Input: part model. Units: mm. Frame: model coordinates. A direction names the side the tool comes from. Give positions to 0.01 mm unless a question says otherwise; leave off trailing zeros. Loops run counter-clockwise (first coordinate to the right, second up) from the corner with the lowest first, then second, coordinate; pieces in that order, holes last. Notation, with made-up numbers: M 71.25,11 L 79.25,11 A29 cw 79.25,41 Z; hole C -24.5,31.25 d1. An arc over 180 degrees is marked long. Return JSON: item names as keys, results as strings. Group by question number.
```python
from build123d import *

# Parameters (mm, degrees)
SKETCH1_W                    = 101.6
SKETCH1_H                    = 101.6
EXTRUDE1_DEPTH               = 3.175
SKETCH2_W                    = 101.6
SKETCH2_H                    = 60.96
EXTRUDE2_DEPTH               = 6.35
EXTRUDE3_DEPTH               = 114.990901501
SKETCH4_W                    = 88.9
SKETCH4_H                    = 66.294
EXTRUDE4_DEPTH               = 35.56
SKETCH5_W                    = 27.305
SKETCH5_H                    = 56.134
EXTRUDE5_DEPTH               = 112.536082502
SKETCH6_W                    = 3.175
SKETCH6_H                    = 56.134
EXTRUDE6_DEPTH               = 12.7
SKETCH7_W                    = 8.89
SKETCH7_H                    = 1.27
EXTRUDE7_DEPTH               = 79.375
SKETCH8_W                    = 5.08
SKETCH8_H                    = 35.814
EXTRUDE8_DEPTH               = 19.558
F_5_16_CLEARANCE_HOLE1_D     = 8.4328
F_5_16_CLEARANCE_HOLE1_DEPTH = 12.954
F_5_16_CLEARANCE_HOLE1_TIP   = 2.533468714
EXTRUDE9_DEPTH               = 6.604
F_8_CLEARANCE_HOLE1_D        = 4.4958
LPATTERN1_COUNT              = 2
LPATTERN1_PITCH              = 10.16


with BuildPart() as part:
    # Sketch1 → Extrude1 (new body)
    with BuildSketch(Plane.XY):
        Rectangle(SKETCH1_W, SKETCH1_H)
    extrude(amount=EXTRUDE1_DEPTH)

    # Sketch2 → Extrude2 (add)
    with BuildSketch(Plane.XY.offset(3.175)):
        Rectangle(SKETCH2_W, SKETCH2_H)
    extrude(amount=EXTRUDE2_DEPTH)

    # Sketch3 → Extrude3 (cut, through all)
    with BuildSketch(Plane(origin=(50.8, 0, 0), x_dir=(0, 0, -1), z_dir=(1, 0, 0))):
        Polygon((-9.525, -17.78), (-4.445, -20.712939367), (-4.445, 20.712939367), (-9.525, 17.78), align=None)
    extrude(amount=-EXTRUDE3_DEPTH, mode=Mode.SUBTRACT)

    # Sketch4 → Extrude4 (add)
    with BuildSketch(Plane(origin=(0, 0, 0), x_dir=(-1, 0, 0), z_dir=(0, 0, -1))):
        with Locations((2.54, 0)):
            Rectangle(SKETCH4_W, SKETCH4_H)
    extrude(amount=EXTRUDE4_DEPTH)

    # Sketch5 → Extrude5 (cut, through all)
    with BuildSketch(Plane(origin=(41.91, 0, 0), x_dir=(0, 0, -1), z_dir=(1, 0, 0))):
        with Locations((16.8275, 0)):
            Rectangle(SKETCH5_W, SKETCH5_H)
    extrude(amount=-EXTRUDE5_DEPTH, mode=Mode.SUBTRACT)

    # Sketch6 → Extrude6 (add)
    with BuildSketch(Plane(origin=(0, 0, -3.175), x_dir=(-1, 0, 0), z_dir=(0, 0, -1))):
        with Locations((45.4025, 0)):
            Rectangle(SKETCH6_W, SKETCH6_H)
    extrude(amount=EXTRUDE6_DEPTH)

    # Sketch7 → Extrude7 (cut)
    with BuildSketch(Plane(origin=(41.91, 0, 0), x_dir=(0, 0, -1), z_dir=(1, 0, 0))):
        with Locations((19.05, -28.702)):
            Rectangle(SKETCH7_W, SKETCH7_H)
    extrude(amount=-EXTRUDE7_DEPTH, mode=Mode.SUBTRACT)

    # Sketch8 → Extrude8 (cut)
    with BuildSketch(Plane(origin=(41.91, 0, 0), x_dir=(0, 0, -1), z_dir=(1, 0, 0))):
        with Locations((33.02, 0)):
            Rectangle(SKETCH8_W, SKETCH8_H)
    extrude(amount=-EXTRUDE8_DEPTH, mode=Mode.SUBTRACT)

    # 5/16 Clearance Hole1
    with Locations(Plane(origin=(12.8016, -33.147, -20.066), x_dir=(-1, 0, 0), z_dir=(0, -1, 0))):
        with Locations((0, 0)):
            Hole(F_5_16_CLEARANCE_HOLE1_D / 2, depth=F_5_16_CLEARANCE_HOLE1_DEPTH)
            with Locations((0, 0, -(F_5_16_CLEARANCE_HOLE1_DEPTH + F_5_16_CLEARANCE_HOLE1_TIP / 2))):  # 118° drill point
                Cone(0, F_5_16_CLEARANCE_HOLE1_D / 2, F_5_16_CLEARANCE_HOLE1_TIP, mode=Mode.SUBTRACT)

    # Sketch11 → Extrude9 (add)
    with BuildSketch(Plane.XY.offset(4.445)):
        Polygon((50.8, 0), (50.8, -5.715), (44.45, -5.715), (44.45, 5.715), (50.8, 5.715), align=None)
    extrude9 = extrude(amount=EXTRUDE9_DEPTH)

    # #8 Clearance Hole1 (through all)
    with Locations(Plane(origin=(50.8, 0, 7.62), x_dir=(0, 0, 1), z_dir=(1, 0, 0))):
        with Locations((0, 0)):
            f_8_clearance_hole1 = Hole(F_8_CLEARANCE_HOLE1_D / 2)

    # LPattern1: Extrude9, #8 Clearance Hole1 ×2
    with Locations(*[(-i * LPATTERN1_PITCH, 0, 0) for i in range(1, LPATTERN1_COUNT)]):
        add(extrude9)
        add(f_8_clearance_hole1, mode=Mode.SUBTRACT)


solid = part.part
```
Item 1: Reachability of faces 4 (the face through (0.711, -19.226, 7.021)), 5 (the face through (-1, -40, 3.175)), 6 (the face through (22.352, 0, -33)), 7 (the face through (-2, 28.067, -17)) from +Z, -Z, +X, -X, +Y, -Y: full face, straight path, thin tool, end or side. Return the list, or none.
Item 2: Section C-C, the plane z = 7.62. Return loops of the section in (x, y) (3 decimals).
Item 3: Section A-A, the plane y = 4. Return loops of the section in (x, z) (3 decimals).
Item 4: Pull-direction query (Z, two-part tool) for faces 1 (the face through (3, -29.337, -19)), 2 (the face through (38, 0, 11.049)), 3 (the face through (37, 5.715, 8)); classes: pulls with the +Z half, pulls with the -Z half, needs draft (parallel to the pull), parting line crosses it, or undercut.
Item 5: Section D-D, the plane x = 30. Return loops of the section in (y, z) (3 decimals), then the cut area to 3 significant figures.
Item 6: Material intervals for line 1 (Z direction, x = 34, y = 23) (3 decimals); line 2 (Y direction, x = -18.5, z = -4); line 3 (Y direction, x = 38.5, z = 7.62) (3 decimals), sorted ascending. Write a range as from..to.
Item 7: First-contact query: pin 1 Ø1.9 at (x, z) = (37, 9) entering from +Y; pin 2 Ø22.5 at (x, y) = (22, 40.5) entering from +Z (3 decimals); pin 3 Ø3 at (x, z) = (36, 6.5) entering from -Y. Flat tips, straight axial feed; report the tip coordinate or a pass-through.
Item 8: Section B-B, the plane x = -13.5. Return loops of the section in (y, z) (3 decimals), then the cut area to 3 significant figures.
Answer below:
{
 "1": {"face 4": "+X, -X", "face 5": "+Z, +X, -X, -Y", "face 6": "-Z, +X", "face 7": "+X"},
 "2": {"outline": "M -50.8,-30.48 L 50.8,-30.48 L 50.8,-18.88 L -50.8,-18.88 Z; M -50.8,18.88 L 50.8,18.88 L 50.8,30.48 L -50.8,30.48 Z; M 34.29,-5.715 L 40.64,-5.715 L 40.64,-2.248 L 34.29,-2.248 Z; M 34.29,2.248 L 40.64,2.248 L 40.64,5.715 L 34.29,5.715 Z; M 44.45,-5.715 L 50.8,-5.715 L 50.8,-2.248 L 44.45,-2.248 Z; M 44.45,2.248 L 50.8,2.248 L 50.8,5.715 L 44.45,5.715 Z"},
 "3": {"outline": "M -50.8,0 L -46.99,0 L -46.99,-15.875 L -43.815,-15.875 L -43.815,-3.175 L 41.91,-3.175 L 41.91,0 L 50.8,0 L 50.8,11.049 L 44.45,11.049 L 44.45,4.445 L 40.64,4.445 L 40.64,11.049 L 34.29,11.049 L 34.29,4.445 L -50.8,4.445 Z; M -46.99,-35.56 L 22.352,-35.56 L 22.352,-30.48 L -46.99,-30.48 Z"},
 "4": {"face 1": "undercut", "face 2": "pulls with the +Z half", "face 3": "needs draft"},
 "5": {"outline": "M -50.8,0 L -33.147,0 L -33.147,-35.56 L -17.907,-35.56 L -17.907,-30.48 L -28.067,-30.48 L -28.067,-23.495 L -29.337,-23.495 L -29.337,-14.605 L -28.067,-14.605 L -28.067,-3.175 L 28.067,-3.175 L 28.067,-30.48 L 17.907,-30.48 L 17.907,-35.56 L 33.147,-35.56 L 33.147,0 L 50.8,0 L 50.8,3.175 L 30.48,3.175 L 30.48,9.525 L 17.78,9.525 L 20.713,4.445 L -20.713,4.445 L -17.78,9.525 L -30.48,9.525 L -30.48,3.175 L -50.8,3.175 Z", "area": "1,150 mm^2"},
 "6": {"line 1": "-35.56..-30.48, -3.175..9.525", "line 2": "-33.15..-28.07, 28.07..33.15", "line 3": "-30.48..-18.88, -5.715..-2.248, 2.248..5.715, 18.88..30.48"},
 "7": {"pin 1": "y = 30.48", "pin 2": "z = 9.525", "pin 3": "y = -30.48"},
 "8": {"outline": "M -50.8,0 L -33.147,0 L -33.147,-35.56 L 33.147,-35.56 L 33.147,0 L 50.8,0 L 50.8,3.175 L 30.48,3.175 L 30.48,9.525 L 17.78,9.525 L 20.713,4.445 L -20.713,4.445 L -17.78,9.525 L -30.48,9.525 L -30.48,3.175 L -50.8,3.175 Z; hole M -29.337,-23.495 L -28.067,-23.495 L -28.067,-30.48 L 28.067,-30.48 L 28.067,-3.175 L -28.067,-3.175 L -28.067,-14.605 L -29.337,-14.605 Z", "area": "1,330 mm^2"}
}
